from build123d import *

# Parameters (mm, degrees)
SKETCH3_OUTSIDE_W               = 25.774
SKETCH3_OUTSIDE_H               = 25.774
CUT_EXTRUDE1_DEPTH              = 48.359986768
F_1_4_0_25_DIAMETER_HOLE1_D     = 6.35
F_1_4_0_25_DIAMETER_HOLE1_DEPTH = 8.7376
F_1_4_0_25_DIAMETER_HOLE1_TIP   = 1.907732465
CHAMFER1_SIZE                   = 0.508
BOSS_EXTRUDE1_START             = -14.986
SKETCH7_R                       = 3.175
BOSS_EXTRUDE1_DEPTH             = 14.986
FILLET1_R                       = 0.508


with BuildPart() as part:
    # Sketch2 → Revolve1 (revolve)
    with BuildSketch(Plane(origin=(0, 0, 0), x_dir=(0, 0, -1), z_dir=(1, 0, 0)), mode=Mode.PRIVATE) as revolve1_sk:
        Polygon((-23.1775, 0), (23.1775, 0), (23.1775, 4.7625), (22.6695, 4.7625), (14.7701, 4.7625), (14.7701, 6.862299966), (-20.9169, 6.862299966), (-20.9169, 5.8928), (-21.9075, 5.8928), (-21.9075, 6.35), (-23.1775, 6.35), align=None)
    revolve(revolve1_sk.sketch.rotate(Axis((0, 0, 23.1775), (0, 0, -1)), 90), axis=Axis((0, 0, 23.1775), (0, 0, -1)))

    # Sketch3 outside → Cut-Extrude1 (cut, through all)
    with BuildSketch(Plane.XY.offset(23.1775)):
        Rectangle(SKETCH3_OUTSIDE_W, SKETCH3_OUTSIDE_H)
        Polygon((7.26292966, -1.38571412), (4.83152846, 5.597024532), (-2.4314012, 6.982738652), (-7.26292966, 1.38571412), (-4.83152846, -5.597024532), (2.4314012, -6.982738652), align=None, mode=Mode.SUBTRACT)
    extrude(amount=-CUT_EXTRUDE1_DEPTH, mode=Mode.SUBTRACT)

    # 1/4 (0.25) Diameter Hole1
    with Locations(Plane(origin=(0, 0, -23.1775), x_dir=(-1, 0, 0), z_dir=(0, 0, -1))):
        with Locations((0, 0)):
            Hole(F_1_4_0_25_DIAMETER_HOLE1_D / 2, depth=F_1_4_0_25_DIAMETER_HOLE1_DEPTH)
            with Locations((0, 0, -(F_1_4_0_25_DIAMETER_HOLE1_DEPTH + F_1_4_0_25_DIAMETER_HOLE1_TIP / 2))):  # 118° drill point
                Cone(0, F_1_4_0_25_DIAMETER_HOLE1_D / 2, F_1_4_0_25_DIAMETER_HOLE1_TIP, mode=Mode.SUBTRACT)

    # Chamfer1
    chamfer1_edges = [part.edges().sort_by_distance(p)[0] for p in [
        (-4.7625, 0, -23.1775),
        (-6.35, 0, 23.1775),
    ]]
    chamfer(chamfer1_edges, length=CHAMFER1_SIZE)

    # Sketch7 → Boss-Extrude1 (add)
    with BuildSketch(Plane(origin=(0, 0, -14.7701), x_dir=(-1, 0, 0), z_dir=(0, 0, -1)).offset(BOSS_EXTRUDE1_START)):
        Polygon((-4.83152846, 5.597024532), (-7.26292966, -1.38571412), (-2.4314012, -6.982738652), (4.83152846, -5.597024532), (7.26292966, 1.38571412), (2.4314012, 6.982738652), align=None)
        Circle(SKETCH7_R, mode=Mode.SUBTRACT)
    extrude(amount=BOSS_EXTRUDE1_DEPTH)

    # Fillet1
    fillet1_edges = [part.edges().sort_by_distance(p)[0] for p in [
        (2.4314012, -6.982738652, -7.2771),
        (-4.83152846, -5.597024532, -7.2771),
        (-7.26292966, 1.38571412, -7.2771),
        (-2.4314012, 6.982738652, -7.2771),
        (7.26292966, -1.38571412, -7.2771),
        (4.83152846, 5.597024532, -7.2771),
    ]]
    fillet(fillet1_edges, radius=FILLET1_R)


solid = part.part
Here's how the part is built. I have some questions about the finished solid (model axes, mm). A direction names the side the tool comes from. Coordinates: 2 decimals unless noted, no trailing zeros. Order: outer loops, then holes, each group sorted by start corner. A loop starts at its lowest first (then second) coordinate and runs counter-clockwise, first axis right, second up.
Item 1: If we section it at A-A on z = -2.5: List the corners of the cut face in (x, y) for me, plus the area to 3 significant figures.
Result sheet:
outline: (-7.17, 1.11) - (-4.93, -5.32) arc R0.51 ccw to (-4.54, -5.65) - (2.14, -6.93) arc R0.51 ccw to (2.62, -6.76) - (7.07, -1.61) arc R0.51 ccw to (7.17, -1.11) - (4.93, 5.32) arc R0.51 ccw to (4.54, 5.65) - (-2.14, 6.93) arc R0.51 ccw to (-2.62, 6.76) - (-7.07, 1.61) arc R0.51 ccw to start
area: 142 mm2
Item 2: If we mould it in two halves opening along Z, with no side actions, what happens to faces 5 (the face through (0.12, -0.538, -12.863)), 6 (the face through (-0.767, -5.843, 21.419)), 7 (the face through (6.03, 2.15, 3.32))? For each: +Z half, -Z half, draft (parallel to the pull), parting line (faces both ways), or undercut.
Result sheet:
face 5: -Z half
face 6: undercut
face 7: draft
Item 3: I need wall thicknesses on line 1 (Y direction, x = 0, z = -21) (1 decimal); line 2 (Z direction, x = 2, y = -5.5); line 3 (Z direction, x = -0.75, y = -6). Which ranges of each line are inside material? Lowest first, please.
Result sheet:
line 1: y = -4.8 to -3.2, 3.2 to 4.8
line 2: z = -14.77 to 23.17
line 3: z = -14.77 to 20.92, 21.91 to 22.97
Item 4: For P1, Ø8, axis at y = -0.5, z = 17.5, coming from the -X side; P2, Ø6, axis at y = 4.5, z = 8.5, coming from the -X side; P3, Ø4, axis at x = -5.5, y = -2.5, coming from the +Z side; P4, Ø1.5, axis at x = -5.5, z = 4.5, coming from the -Y side, each with a flat end and sliding along its axis, tell me the tip position at first contact or that it passes through.
Result sheet:
P1: stops at x = -6.86
P2: stops at x = -6.7
P3: stops at z = 23.18
P4: stops at y = -4.95
Item 5: If we section it at C-C on z = 4: List the corners of the cut face in (x, y) for me.
Result sheet:
outline: (-6.86, 0.22) - (-5.24, -4.44) arc R6.86 ccw to (-3.62, -5.83) - (1.22, -6.75) arc R6.86 ccw to (3.23, -6.05) - (6.46, -2.32) arc R6.86 ccw to (6.86, -0.22) - (5.24, 4.44) arc R6.86 ccw to (3.62, 5.83) - (-1.22, 6.75) arc R6.86 ccw to (-3.23, 6.05) - (-6.46, 2.32) arc R6.86 ccw to start
Item 6: If we section it at B-B on z = -14: List the corners of the cut face in (x, y) for me, plus the area to 3 significant figures.
Result sheet:
outline: (-7.17, 1.11) - (-4.93, -5.32) arc R0.51 ccw to (-4.54, -5.65) - (2.14, -6.93) arc R0.51 ccw to (2.62, -6.76) - (7.07, -1.61) arc R0.51 ccw to (7.17, -1.11) - (4.93, 5.32) arc R0.51 ccw to (4.54, 5.65) - (-2.14, 6.93) arc R0.51 ccw to (-2.62, 6.76) - (-7.07, 1.61) arc R0.51 ccw to start; hole circle Ø4.89 at (0, 0)
area: 123 mm2
Item 7: For faces 1 (the face through (-1, 6, 20.917)), 2 (the face through (-5, 0, -14.77)), 3 (the face through (2.271, -6.476, 10.711)), 4 (the face through (-4.6, -5.3, 0.216)), which set-ups out of +Z, -Z, +X, -X, +Y, -Y let a thin tool reach every point of the face, with its end or its side?
Result sheet:
face 1: none
face 2: -Z
face 3: +Z, +X, -Y
face 4: +Z, -X, -Y
